Source: CAD feature listing. Evaluate the final solid. Frame: model axes, mm. Give positions to 0.01 mm unless a question says otherwise; leave off trailing zeros. Order: outer loops, then holes, each group sorted by start corner. A loop starts at its lowest first (then second) coordinate and runs counter-clockwise, first axis right, second up.
1) Section A-A, the plane x = -2.54. Return loops of the section in (y, z), plus the area to 3 significant figures.
2) First-contact query: P1, Ø2.5, axis at x = -55.626, z = -26.67, coming from the +Y side. Flat tip, straight axial feed; report the tip coordinate or a pass-through.
3) Section C-C, the plane y = 0.45. Return loops of the section in (x, z), plus the area to 3 significant figures.
4) Material intervals for line 1 (X direction, y = 0.8, z = -26.67); line 2 (Z direction, x = -2.54, y = 0.3); line 3 (X direction, y = 1.4, z = -26.25), sorted ascending.
5) Section B-B, the plane z = -26.67. Return loops of the section in (x, y).
Autodesk Inventor part; units mm, degrees
ref_plane "YZ Plane" through (0, 0, 0) normal (1, 0, 0) x (0, 1, 0)
ref_plane "XZ Plane" through (0, 0, 0) normal (0, 1, 0) x (-1, 0, 0)
ref_plane "XY Plane" through (0, 0, 0) normal (0, 0, 1) x (1, 0, 0)
sketch "Sketch1" plane through (0, 0, 0) normal (0, 1, 0) x (-1, 0, 0)
  line L0 (0, 0) -> (58.166, 0)
  line L1 (58.166, 0) -> (58.166, -29.21)
  line L2 (58.166, -29.21) -> (0, -29.21)
  line L3 (0, -29.21) -> (0, 0)
  dimension "d0" = 58.166
  dimension "d1" = 29.21
extrude "Extrusion1" add sketch "Sketch1" along normal blind 1.5748
hole "Hole1" at (-55.626, 1.5748, -2.54) direction (0, -1, 0) diameter 3.048 depth 25.4 tip angle 118
hole "Hole2" at (-55.626, 1.5748, -26.67) direction (0, -1, 0) diameter 3.048 depth 25.4 tip angle 118
hole "Hole3" at (-2.54, 1.5748, -26.67) direction (0, -1, 0) diameter 3.048 depth 25.4 tip angle 118
hole "Hole4" at (-2.54, 1.5748, -2.54) direction (0, -1, 0) diameter 3.048 depth 25.4 tip angle 118
properties part number "firebeetle_board"
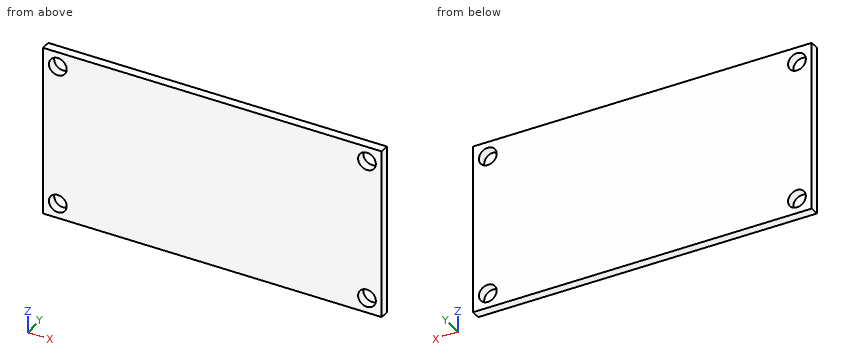
From the geometry:
1. outline: (0, -29.21) - (1.57, -29.21) - (1.57, -28.19) - (0, -28.19) - close; (0, -25.15) - (1.57, -25.15) - (1.57, -4.06) - (0, -4.06) - close; (0, -1.02) - (1.57, -1.02) - (1.57, 0) - (0, 0) - close
1. area: 36.4 mm2
2. P1: passes through
3. outline: (-58.17, -29.21) - (0, -29.21) - (0, 0) - (-58.17, 0) - close; hole circle Ø3.05 at (-55.63, -26.67); hole circle Ø3.05 at (-55.63, -2.54); hole circle Ø3.05 at (-2.54, -26.67); hole circle Ø3.05 at (-2.54, -2.54)
3. area: 1,670 mm2
4. line 1: x = -58.17 to -57.15, -54.1 to -4.06, -1.02 to 0
4. line 2: z = -29.21 to -28.19, -25.15 to -4.06, -1.02 to 0
4. line 3: x = -58.17 to -57.09, -54.16 to -4, -1.08 to 0
5. outline: (-58.17, 0) - (-57.15, 0) - (-57.15, 1.57) - (-58.17, 1.57) - close; (-54.1, 0) - (-4.06, 0) - (-4.06, 1.57) - (-54.1, 1.57) - close; (-1.02, 0) - (0, 0) - (0, 1.57) - (-1.02, 1.57) - close
